Build history of the part. All positions in model axes, mm. Give positions to 0.01 mm unless a question says otherwise; leave off trailing zeros. Order: outer loops, then holes, each group sorted by start corner. A loop starts at its lowest first (then second) coordinate and runs counter-clockwise, first axis right, second up. Notation, with made-up numbers: (46, 12.5) -> (78, 12.5) arc R36 cw to (78, 46.5) -> close; hole circle Ø2 at (-22.5, 72.25). An arc over 180 degrees is marked (long way). One line per item, written item: value. Start each with the question number.
(1) Pin check, flat tips, straight feed: pin 1 (3 mm diameter, centred on y = 11, z = 5, fed in from +X); pin 2 (1.5 mm diameter, centred on y = 0, z = 3.5, fed in from +X). Stop position of each tip, or through.
(2) Probe line 1 (X direction, y = 12.75, z = 3.5); line 2 (Z direction, x = 3.25, y = -5.5); line 3 (Y direction, x = -2.5, z = 2). List the from-to ranges inside material, lowest first.
(3) Saw through at C-C on z = 3.75. Give the cut face in (x, y).
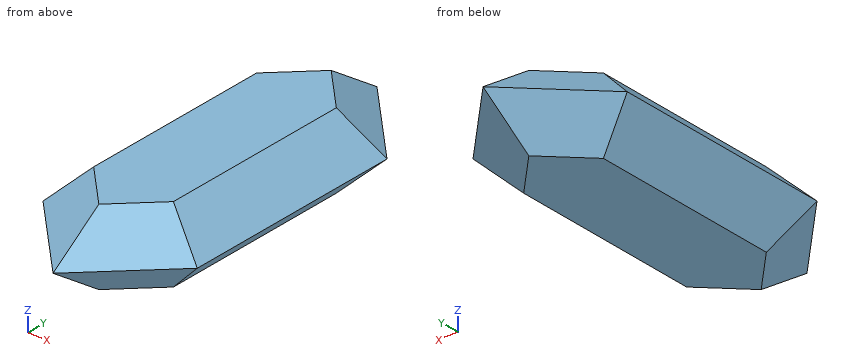
```python
from build123d import *

# Parameters (mm, degrees)
F1_DEPTH = 6
F2_SIZE  = 2.99999


# Not quite as in the source:
# - a fillet or chamfer is up to 0.001 mm smaller than in the source, because OpenCascade refuses the exact size


with BuildPart() as f1:
    # F0 (on Top) → F1 (new body)
    with BuildSketch(Plane.XY):
        Polygon((-6.2132034356, 8.7867965644), (-6.2132034356, 0), (-6.2132034356, -8.7867965644), (0, -15), (6.2132034356, -8.7867965644), (6.2132034356, 0), (6.2132034356, 8.7867965644), (0, 15), align=None)
    extrude(amount=F1_DEPTH)

    # F2 (size 3 in the source; OpenCascade refuses exactly that, so slightly less here)
    f2_edges = [f1.edges().sort_by_distance(p)[0] for p in [
        (-3.106602, 11.893398, 6),
        (3.106602, 11.893398, 6),
        (6.213203, 0, 6),
        (-6.213203, 0, 6),
        (-3.106602, -11.893398, 6),
        (3.106602, -11.893398, 6),
        (-3.106602, 11.893398, 0),
        (-6.213203, 0, 0),
        (-3.106602, -11.893398, 0),
        (3.106602, -11.893398, 0),
        (6.213203, 0, 0),
        (3.106602, 11.893398, 0),
    ]]
    chamfer(f2_edges, length=F2_SIZE)


solid = f1.part
```
Results below:
1. pin 1: stops at x = 3.77
1. pin 2: stops at x = 6.21
2. line 1: x = -1.54 to 1.54
2. line 2: z = 0.04 to 5.96
2. line 3: y = -11.09 to 11.09
3. outline: (-5.46, -8.48) -> (0, -13.94) -> (5.46, -8.48) -> (5.46, 8.48) -> (0, 13.94) -> (-5.46, 8.48) -> close
